from build123d import *

# Parameters (mm, degrees)
SKETCH1_W                = 171
SKETCH1_H                = 104.5
SKETCH1_W_2              = 155
SKETCH1_H_2              = 88
BOSS_EXTRUDE1_DEPTH      = 1
SKETCH2_W                = 171
SKETCH2_H                = 104.5
SKETCH2_W_2              = 167
SKETCH2_H_2              = 100.5
BOSS_EXTRUDE2_DEPTH      = 4
SKETCH3_W                = 35
SKETCH3_H                = 8.699372258
CUT_EXTRUDE1_DEPTH       = 14
BOSS_EXTRUDE3_DEPTH      = 16
BOSS_EXTRUDE3_DEPTH_BACK = 1
SKETCH4_W                = 7
SKETCH4_H                = 19.695550369
FILLET1_R                = 12
CHAMFER1_SIZE            = 30
CHAMFER1_SIZE_2          = 5
FILLET2_R                = 8
SKETCH5_R                = 1.75
CUT_EXTRUDE2_DEPTH       = 216


with BuildPart() as part:
    # Sketch1 → Boss-Extrude1 (new body)
    with BuildSketch(Plane(origin=(0, 0, 0), x_dir=(1, 0, 0), z_dir=(0, 1, 0))):
        with Locations((0, -1.75)):
            Rectangle(SKETCH1_W, SKETCH1_H)
        Rectangle(SKETCH1_W_2, SKETCH1_H_2, mode=Mode.SUBTRACT)
    extrude(amount=BOSS_EXTRUDE1_DEPTH)

    # Sketch2 → Boss-Extrude2 (add)
    with BuildSketch(Plane(origin=(0, 1, 0), x_dir=(1, 0, 0), z_dir=(0, 1, 0))):
        with Locations((0, -1.75)):
            Rectangle(SKETCH2_W, SKETCH2_H)
        with Locations((0, -1.75)):
            Rectangle(SKETCH2_W_2, SKETCH2_H_2, mode=Mode.SUBTRACT)
    extrude(amount=BOSS_EXTRUDE2_DEPTH)

    # Sketch3 → Cut-Extrude1 (cut)
    with BuildSketch(Plane(origin=(0, 1, 0), x_dir=(1, 0, 0), z_dir=(0, 1, 0))):
        with Locations((0, -52)):
            Rectangle(SKETCH3_W, SKETCH3_H)
    extrude(amount=CUT_EXTRUDE1_DEPTH, mode=Mode.SUBTRACT)

    # Sketch4 → Boss-Extrude3 (add, two sides: drawn at the far end of the back side and taken through both)
    with BuildSketch(Plane(origin=(0, 1, 0), x_dir=(1, 0, 0), z_dir=(0, 1, 0)).offset(-BOSS_EXTRUDE3_DEPTH_BACK)):
        with Locations((-87, -44.152224816)):
            Rectangle(SKETCH4_W, SKETCH4_H)
        with Locations((87, -44.152224816)):
            Rectangle(SKETCH4_W, SKETCH4_H)
    extrude(amount=BOSS_EXTRUDE3_DEPTH + BOSS_EXTRUDE3_DEPTH_BACK)

    # Fillet1
    fillet1_edges = [part.edges().sort_by_distance(p)[0] for p in [
        (87, 17, 34.304449631),
        (-87, 17, 34.304449631),
    ]]
    fillet(fillet1_edges, radius=FILLET1_R)

    # Chamfer1
    # the kernel refuses this chamfer: 30, 5 mm, written as the material it adds along each edge
    with BuildSketch(Plane(origin=(85.5, 5, 34.304449631), x_dir=(-0.006326222023777661, 0, -0.999979989257238), z_dir=(0, -1, 0))) as chamfer1_piece_1_section:
        Polygon((CHAMFER1_SIZE * 0.999979989257, CHAMFER1_SIZE * 0.00632622202378), (-CHAMFER1_SIZE_2 * 0.00632622202378, CHAMFER1_SIZE_2 * 0.999979989257), (0, 0), align=None)
    chamfer1_piece_1 = extrude(amount=5, mode=Mode.PRIVATE)
    chamfer1_piece_1 = split(chamfer1_piece_1, bisect_by=Plane(origin=(90.5, 2.5, 23.467018092), z_dir=(-1, 0, 0)), keep=Keep.TOP, mode=Mode.PRIVATE)
    add(chamfer1_piece_1)
    with BuildSketch(Plane(origin=(-85.5, 0, 34.304449631), x_dir=(0.006326222023777661, 0, -0.999979989257238), z_dir=(0, 1, 0))) as chamfer1_piece_2_section:
        Polygon((CHAMFER1_SIZE * 0.999979989257, CHAMFER1_SIZE * 0.00632622202378), (-CHAMFER1_SIZE_2 * 0.00632622202378, CHAMFER1_SIZE_2 * 0.999979989257), (0, 0), align=None)
    chamfer1_piece_2 = extrude(amount=5, mode=Mode.PRIVATE)
    chamfer1_piece_2 = split(chamfer1_piece_2, bisect_by=Plane(origin=(-90.5, 2.5, 23.467018092), z_dir=(1, 0, 0)), keep=Keep.TOP, mode=Mode.PRIVATE)
    add(chamfer1_piece_2)

    # Fillet2
    fillet2_edges = [part.edges().sort_by_distance(p)[0] for p in [
        (87, 17, 54),
        (-87, 17, 54),
    ]]
    fillet(fillet2_edges, radius=FILLET2_R)

    # Sketch5 → Cut-Extrude2 (cut)
    with BuildSketch(Plane.ZY.offset(90.5)):
        with Locations((44.152224816, 9.892685603)):
            Circle(SKETCH5_R)
    extrude(amount=-CUT_EXTRUDE2_DEPTH, mode=Mode.SUBTRACT)


solid = part.part
Design review of the part built by this model. Coordinates are the model's own, in mm. A direction names the side the tool comes from. Coordinates: 2 decimals unless noted, no trailing zeros. Loops run counter-clockwise (first coordinate to the right, second up) from the corner with the lowest first, then second, coordinate; pieces in that order, holes last. Notation, with made-up numbers: (-15.75, 30.25) - (29.25, 30.25) arc R26 ccw to (29.25, 48.25) - close; hole circle Ø2 at (-31, 33). An arc over 180 degrees is marked (long way). Use CSV: the item, a comma, the result in double quotes. Start each with the question number.
1. Add section A-A on x = -12. Give the boundary of the cut face in (y, z), plus the area to 3 significant figures.
2. Clearance check with flat-ended pins moving along their axes: pin 1 (2 mm diameter, centred on x = -50, z = 53, fed in from +Y); pin 2 (1.1 mm diameter, centred on y = 0.5, z = -7.5, fed in from -X); pin 3 (4 mm diameter, centred on y = 1.5, z = -35, fed in from +X). State where each tip first meets the part, or that it passes through.
3. For faces 1 (the flat face through (-85.5, 2, -23)), 2 (the flat face through (85.5, 2, -23)), 3 (the flat face through (-90.5, 6, 44)), 4 (the flat face through (0, 5, -49)), 5 (the flat face through (83.5, 4, 15)), list the 3-axis set-ups (+Z, -Z, +X, -X, +Y, -Y) from which the entire face can be reached by the end or side of a thin tool; tool diameter is ignored.
4. To check wall thickness, follow probe 1 along Z at (x, y) = (39, 1.5); probe 2 along Z at (x, y) = (-4.5, 0.5); probe 3 along X at (y, z) = (4, -10.5). State the ranges of each line that lie inside material, in increasing order.
5. Mouldability with a two-part tool opening along X and no side actions: class faces 6 (the cylindrical face through (-87.049, 9.222, 45.769)), 7 (the flat face through (-0.4, 1, 44.3)), 8 (the flat face through (87.965, 2.535, 19.094)) as released by +X, released by -X, zero draft, split by the parting line, or undercut.
6. Add section B-B on z = -3. Give the boundary of the cut face in (x, y).
7. Add section D-D on x = 19.5. Give the boundary of the cut face in (y, z).
8. Add section C-C on y = 3.25. Give the boundary of the cut face in (x, z), plus the area to 3 significant figures.
Resolved:
1,outline,"(0, -50.5) - (5, -50.5) - (5, -48.5) - (1, -48.5) - (1, -44) - (0, -44) - close; (0, 44) - (1, 44) - (1, 54) - (0, 54) - close"
1,area,"24.5 mm2"
2,pin 1,"y = 5"
2,pin 2,"x = -85.5"
2,pin 3,"x = 85.5"
3,face 1,"-Z, -X, +Y, -Y"
3,face 2,"-Z, +X, +Y, -Y"
3,face 3,"+Z, -Z, -X, +Y, -Y"
3,face 4,"-Z, +X, -X, +Y"
3,face 5,"+Y"
4,probe 1,"-50.5 to -48.5, 52 to 54"
4,probe 2,"-50.5 to -44, 44 to 54"
4,probe 3,"-85.5 to -83.5, 83.5 to 85.5"
5,face 6,"zero draft"
5,face 7,"undercut"
5,face 8,"released by +X"
6,outline,"(-85.5, 0) - (-77.5, 0) - (-77.5, 1) - (-83.5, 1) - (-83.5, 5) - (-85.5, 5) - close; (77.5, 0) - (85.5, 0) - (85.5, 5) - (83.5, 5) - (83.5, 1) - (77.5, 1) - close"
7,outline,"(0, -50.5) - (5, -50.5) - (5, -48.5) - (1, -48.5) - (1, -44) - (0, -44) - close; (0, 44) - (1, 44) - (1, 52) - (5, 52) - (5, 54) - (0, 54) - close"
8,outline,"(-90.5, 34.3) - (-85.5, 4.3) - (-85.5, -50.5) - (85.5, -50.5) - (85.5, 4.3) - (90.5, 34.3) - (90.5, 54) - (17.5, 54) - (17.5, 52) - (83.5, 52) - (83.5, -48.5) - (-83.5, -48.5) - (-83.5, 52) - (-17.5, 52) - (-17.5, 54) - (-90.5, 54) - close"
8,area,"1,360 mm2"
